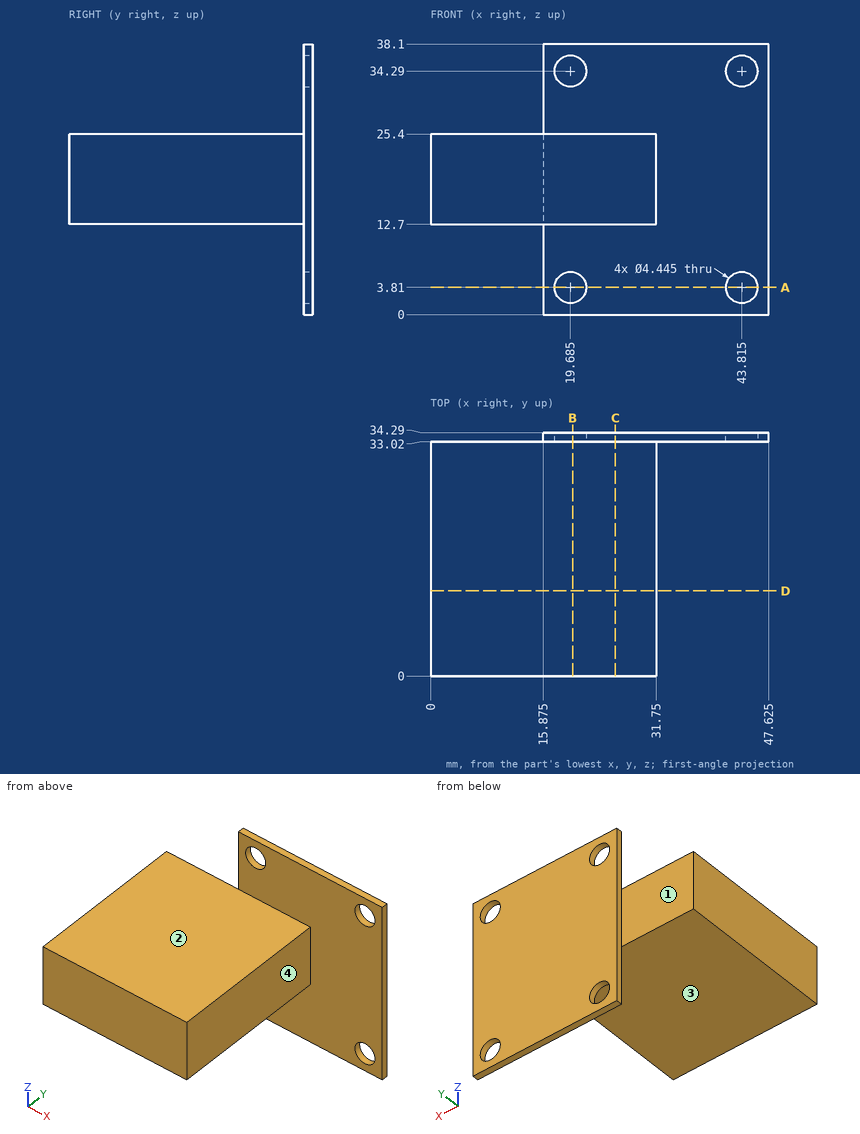
Part print with two shaded views. Sizes in mm from the minimum x, y, z corner. A direction names the side the tool comes from. Round coordinates to 2 decimals unless told otherwise and drop trailing zeros. Write each loop counter-clockwise with the first axis right and the second up, starting at its lowest first coordinate (ties: lowest second). Pieces come first, ordered by that corner, then holes. Notation, with made-up numbers: (65.5, -6) -> (70.5, -6) arc R18 cw to (70.5, 5) -> close; hole circle Ø10 at (61.25, 60.25). An arc over 180 degrees is marked (long way). Put each result on its own line as item: value.
Item 1: Tool access for the marked faces 1, 2, 3 and 4: list every direction of +Z, -Z, +X, -X, +Y, -Y with a clear straight run to the whole face (end or side of a thin tool).
Here are the results:
face 1: +Z, -Z, -X, +Y
face 2: +Z, +X, -X, -Y
face 3: -Z, +X, -X, -Y
face 4: +Z, -Z, +X, -Y
Item 2: Wall check: probe 1 along Z at (x, y) = (27, 6); probe 2 along X at (y, z) = (14, 14); probe 3 along Y at (x, z) = (36.5, 35). Give the ranges that are in metal, low to high. Write a range as from..to.
Here are the results:
probe 1: z = 12.7..25.4
probe 2: x = 0..31.75
probe 3: y = 33.02..34.29
Item 3: Slice it at B-B, the plane x = 20. Give the cut face in (y, z), plus the area to 3 significant figures.
Here are the results:
outline: (0, 12.7) -> (33.02, 12.7) -> (33.02, 6.01) -> (34.29, 6.01) -> (34.29, 32.09) -> (33.02, 32.09) -> (33.02, 25.4) -> (0, 25.4) -> close; (33.02, 0) -> (34.29, 0) -> (34.29, 1.61) -> (33.02, 1.61) -> close; (33.02, 36.49) -> (34.29, 36.49) -> (34.29, 38.1) -> (33.02, 38.1) -> close
area: 457 mm^2
Item 4: Slice it at D-D, the plane y = 12. Give the cut face in (x, z), plus the area to 3 significant figures.
Here are the results:
outline: (0, 12.7) -> (31.75, 12.7) -> (31.75, 25.4) -> (0, 25.4) -> close
area: 403 mm^2
Item 5: Slice it at A-A, the plane z = 3.81. Give the cut face in (x, y) (1 decimal), plus the area to 3 significant figures.
Here are the results:
outline: (15.9, 33) -> (17.5, 33) -> (17.5, 34.3) -> (15.9, 34.3) -> close; (21.9, 33) -> (41.6, 33) -> (41.6, 34.3) -> (21.9, 34.3) -> close; (46, 33) -> (47.6, 33) -> (47.6, 34.3) -> (46, 34.3) -> close
area: 29.0 mm^2
Item 6: Slice it at C-C, the plane x = 26. Give the cut face in (y, z).
Here are the results:
outline: (0, 12.7) -> (33.02, 12.7) -> (33.02, 0) -> (34.29, 0) -> (34.29, 38.1) -> (33.02, 38.1) -> (33.02, 25.4) -> (0, 25.4) -> close
Item 7: Flat gauge pins, fed straight in: P1, Ø6.5, axis at y = 20, z = 16.5, coming from the +X side; P2, Ø4, axis at x = 19.685, z = 34.29, coming from the +Y side; P3, Ø9.5, axis at x = 14, y = 20.5, coming from the -Z side; P4, Ø6.5, axis at x = 5, z = 19, coming from the +Y side. Where does each tip first touch, or does it go through?
Here are the results:
P1: stops at x = 31.75
P2: passes through
P3: stops at z = 12.7
P4: stops at y = 33.02
